Part model, mm, in its own coordinate system. A direction names the side the tool comes from. Coordinates: 2 decimals unless noted, no trailing zeros. Order: outer loops, then holes, each group sorted by start corner. A loop starts at its lowest first (then second) coordinate and runs counter-clockwise, first axis right, second up.
1) Cut at C-C (z = 2). List the corners of the cut face in (x, y).
2) Wall check: L1, parallel to Y at x = 0, z = 4.5; L2, parallel to Y at x = 0, z = 2.3; L3, parallel to X at y = 24, z = 9.5. Give the ranges that are in metal, low to high.
3) Cut at A-A (y = 21.5). List the corners of the cut face in (x, z), and give its area (3 significant figures).
4) Cut at B-B (y = 0). List the corners of the cut face in (x, z).
5) Cut at D-D (x = -7). List the corners of the cut face in (y, z).
6) Mould opens along Z. For faces 1 (the cylindrical face through (0.221, 30.055, 8.521)), 2 (the flat face through (-3, 5, 0)), 3 (the flat face through (0, 23, 7)) say: +Z half, -Z half, draft (parallel to the pull), parting line (faces both ways), or undercut.
7) Tool access for faces 4 (the cylindrical face through (-0.596, -2.685, 3.451)), 5 (the flat face through (-4, 20, 1)), 6 (the flat face through (4, 20, 9)), 7 (the cylindrical face through (0.596, 4.315, 2.712)), 8 (the flat face through (2.2, -2.2, 7)): list every direction of +Z, -Z, +X, -X, +Y, -Y with a clear straight run to the whole face (end or side of a thin tool).
8) Pin check, flat tips, straight feed: pin 1 Ø6 at (y, z) = (27.5, 5.5) entering from +X; pin 2 Ø1.5 at (y, z) = (-5, 2.5) entering from +X; pin 3 Ø1.6 at (x, y) = (0.5, -5.5) entering from -Z. Stop position of each tip, or through.
```python
from build123d import *

# Parameters (mm, degrees)
ESQUISSE1_R             = 13
ESQUISSE1_R_2           = 2.75
ESQUISSE1_R_3           = 1.65
BOSS_EXTRU_1_DEPTH      = 10
ESQUISSE2_R             = 10.5
ENL_V_MAT_EXTRU_1_DEPTH = 3
ESQUISSE3_R             = 2.75
ENL_V_MAT_EXTRU_2_DEPTH = 5.5
ESQUISSE4_R             = 1.7
BOSS_EXTRU_2_DEPTH      = 3
ESQUISSE5_R             = 2
ENL_V_MAT_EXTRU_3_DEPTH = 3


with BuildPart() as part:
    # Esquisse1 → Boss.-Extru.1 (new body)
    with BuildSketch(Plane.XY):
        Circle(ESQUISSE1_R)
        Circle(ESQUISSE1_R_2, mode=Mode.SUBTRACT)
        with Locations((-7, 0)):
            Circle(ESQUISSE1_R_3, mode=Mode.SUBTRACT)
        with Locations((0, 7)):
            Circle(ESQUISSE1_R_3, mode=Mode.SUBTRACT)
        with Locations((7, 0)):
            Circle(ESQUISSE1_R_3, mode=Mode.SUBTRACT)
        with Locations((0, -7)):
            Circle(ESQUISSE1_R_3, mode=Mode.SUBTRACT)
    extrude(amount=BOSS_EXTRU_1_DEPTH)

    # Esquisse2 → Enlèv. mat.-Extru.1 (cut)
    with BuildSketch(Plane.XY.offset(10)):
        Circle(ESQUISSE2_R)
    extrude(amount=-ENL_V_MAT_EXTRU_1_DEPTH, mode=Mode.SUBTRACT)

    # Esquisse3 → Enlèv. mat.-Extru.2 (cut)
    with BuildSketch(Plane(origin=(0, 0, 0), x_dir=(-1, 0, 0), z_dir=(0, 0, -1))):
        with Locations((-7, 0)):
            Circle(ESQUISSE3_R)
        with Locations((0, 7)):
            Circle(ESQUISSE3_R)
        with Locations((7, 0)):
            Circle(ESQUISSE3_R)
        with Locations((0, -7)):
            Circle(ESQUISSE3_R)
    extrude(amount=-ENL_V_MAT_EXTRU_2_DEPTH, mode=Mode.SUBTRACT)

    # Esquisse4 → Boss.-Extru.2 (add)
    with BuildSketch(Plane(origin=(0, 0, 0), x_dir=(-1, 0, 0), z_dir=(0, 0, -1))):
        with BuildLine():
            Line((-4, 28.369316877), (-4, 12.369316877))
            ThreePointArc((-4, 12.369316877), (0, 13), (4, 12.369316877))
            Line((4, 12.369316877), (4, 28.369316877))
            ThreePointArc((4, 28.369316877), (0, 32.369316877), (-4, 28.369316877))
        make_face()
        with Locations((0, 28.369316877)):
            Circle(ESQUISSE4_R, mode=Mode.SUBTRACT)
    boss_extru_2 = extrude(amount=-BOSS_EXTRU_2_DEPTH)

    # Symétrie1: Boss.-Extru.2 across plane
    add(boss_extru_2.mirror(Plane.XY.offset(5)))

    # Esquisse5 → Enlèv. mat.-Extru.3 (cut)
    with BuildSketch(Plane(origin=(0, 0, 0), x_dir=(-1, 0, 0), z_dir=(0, 0, -1))):
        with Locations((0, 28.369316877)):
            Circle(ESQUISSE5_R)
    extrude(amount=-ENL_V_MAT_EXTRU_3_DEPTH, mode=Mode.SUBTRACT)


solid = part.part
```
Geometry check:
1. outline: (-4, 12.37) arc R13 ccw (long way) to (4, 12.37) - (4, 28.37) arc R4 ccw to (-4, 28.37) - close; hole circle Ø5.5 at (-7, 0); hole circle Ø5.5 at (0, -7); hole circle Ø5.5 at (0, 0); hole circle Ø5.5 at (0, 7); hole circle Ø4 at (0, 28.37); hole circle Ø5.5 at (7, 0)
2. L1: y = -13 to -9.75, -4.25 to -2.75, 2.75 to 4.25, 9.75 to 13
2. L2: y = -13 to -9.75, -4.25 to -2.75, 2.75 to 4.25, 9.75 to 26.37, 30.37 to 32.37
2. L3: x = -4 to 4
3. outline: (-4, 0) - (4, 0) - (4, 3) - (-4, 3) - close; (-4, 7) - (4, 7) - (4, 10) - (-4, 10) - close
3. area: 48.0 mm2
4. outline: (-13, 0) - (-9.75, 0) - (-9.75, 5.5) - (-8.65, 5.5) - (-8.65, 7) - (-10.5, 7) - (-10.5, 10) - (-13, 10) - close; (-5.35, 5.5) - (-4.25, 5.5) - (-4.25, 0) - (-2.75, 0) - (-2.75, 7) - (-5.35, 7) - close; (2.75, 0) - (4.25, 0) - (4.25, 5.5) - (5.35, 5.5) - (5.35, 7) - (2.75, 7) - close; (8.65, 5.5) - (9.75, 5.5) - (9.75, 0) - (13, 0) - (13, 10) - (10.5, 10) - (10.5, 7) - (8.65, 7) - close
5. outline: (-10.95, 0) - (-2.75, 0) - (-2.75, 5.5) - (-1.65, 5.5) - (-1.65, 7) - (-7.83, 7) - (-7.83, 10) - (-10.95, 10) - close; (1.65, 5.5) - (2.75, 5.5) - (2.75, 0) - (10.95, 0) - (10.95, 10) - (7.83, 10) - (7.83, 7) - (1.65, 7) - close
6. face 1: draft
6. face 2: -Z half
6. face 3: undercut
7. face 4: +Z, -Z
7. face 5: +Z, -Z, -X, +Y
7. face 6: +Z, -Z, +X, +Y
7. face 7: -Z
7. face 8: +Z
8. pin 1: stops at x = 4
8. pin 2: stops at x = 12.29
8. pin 3: stops at z = 5.5
